Input: part model. Units: mm. Frame: model coordinates. Face numbers are marked on the shaded views. A direction names the side the tool comes from. Give positions to 0.01 mm unless a question says otherwise; leave off trailing zeros. Order: outer loops, then holes, each group sorted by start corner. A loop starts at its lowest first (then second) coordinate and runs counter-clockwise, first axis right, second up. Notation, with made-up numbers: (45, -27.5) - (61, -27.5) arc R21 cw to (61, 8.5) - close; hole circle Ø2 at (86.5, 63). An arc over 180 degrees is marked (long way). Answer in a Markdown table with one row per item. Add a question column.
1. Section query B-B on z = 6. Return loops of the section in (x, y).
2. Mould query, pull axis Z, two halves, no side actions, for the marked faces 1, 2 and 3. Classes: released by +Z, released by -Z, zero draft, split by the parting line, or undercut.
3. Section query D-D on x = 2.75. Return loops of the section in (y, z), and give its area (3 significant figures).
4. Contact query for flat-ended pins moving along their axis: pin 1 (5 mm diameter, centred on x = 4, y = -2.5, fed in from +Z); pin 2 (0.7 mm diameter, centred on x = 1, y = 14.5, fed in from +Z); pin 3 (3.5 mm diameter, centred on x = 12, z = 8.5, fed in from +Y). Output: stop coordinate, or through.
5. Ray query, line 1 (X direction, y = -8.25, z = 1.5); line 2 (Y direction, x = -13.5, z = 3); line 3 (Z direction, x = 6.25, y = 3.5). Return the intervals inside material, ascending. Write a range as [from, to].
6. Access query for the marked faces 4, 5 and 6. Directions: +Z, -Z, +X, -X, +Y, -Y. A direction counts if a zero-diameter tool reaches every point of the face in a straight line with its end or side. Return the directions, or none.
7. Section query C-C on y = -4. Return loops of the section in (x, z), and give its area (3 significant figures).
8. Section query A-A on z = 8.25. Return loops of the section in (x, y).
```python
from build123d import *

# Parameters (mm, degrees)
SKETCH1_W           = 30
SKETCH1_H           = 26
BOSS_EXTRUDE1_DEPTH = 10
CUT_EXTRUDE2_DEPTH  = 3.5
SKETCH3_W           = 3
SKETCH3_H           = 3
CUT_EXTRUDE3_DEPTH  = 3.5
SKETCH4_W           = 28
SKETCH4_H           = 23.6
CUT_EXTRUDE4_DEPTH  = 5.5
SKETCH5_W           = 3.7
SKETCH5_H           = 0.9
BOSS_EXTRUDE2_DEPTH = 1
SKETCH6_W           = 3.7
SKETCH6_H           = 0.9
BOSS_EXTRUDE3_DEPTH = 1


with BuildPart() as part:
    # Sketch1 → Boss-Extrude1 (new body)
    with BuildSketch(Plane.XY):
        with Locations((0.224911006, 2.218978102)):
            Rectangle(SKETCH1_W, SKETCH1_H)
    extrude(amount=BOSS_EXTRUDE1_DEPTH)

    # Sketch2 → Cut-Extrude2 (cut)
    with BuildSketch(Plane.XY.offset(10)):
        with BuildLine():
            Line((-13.775088994, 9.218978102), (-13.775088994, -4.781021898))
            ThreePointArc((-13.775088994, -4.781021898), (-12.896409337, -6.902342241), (-10.775088994, -7.781021898))
            Line((-10.775088994, -7.781021898), (-10.775088994, -10.781021898))
            Line((-10.775088994, -10.781021898), (11.224911006, -10.781021898))
            Line((11.224911006, -10.781021898), (11.224911006, -7.781021898))
            ThreePointArc((11.224911006, -7.781021898), (13.34623135, -6.902342241), (14.224911006, -4.781021898))
            Line((14.224911006, -4.781021898), (14.224911006, 9.218978102))
            ThreePointArc((14.224911006, 9.218978102), (13.34623135, 11.340298446), (11.224911006, 12.218978102))
            Line((11.224911006, 12.218978102), (11.224911006, 15.218978102))
            Line((11.224911006, 15.218978102), (-10.775088994, 15.218978102))
            Line((-10.775088994, 15.218978102), (-10.775088994, 12.218978102))
            ThreePointArc((-10.775088994, 12.218978102), (-12.896409337, 11.340298446), (-13.775088994, 9.218978102))
        make_face()
    extrude(amount=-CUT_EXTRUDE2_DEPTH, mode=Mode.SUBTRACT)

    # Sketch3 → Cut-Extrude3 (cut)
    with BuildSketch(Plane.XY.offset(10)):
        with Locations((-12.275088994, 13.718978102)):
            Rectangle(SKETCH3_W, SKETCH3_H)
        with Locations((12.724911006, -9.281021898)):
            Rectangle(SKETCH3_W, SKETCH3_H)
        with Locations((-12.275088994, -9.281021898)):
            Rectangle(SKETCH3_W, SKETCH3_H)
        with Locations((12.724911006, 13.718978102)):
            Rectangle(SKETCH3_W, SKETCH3_H)
    extrude(amount=-CUT_EXTRUDE3_DEPTH, mode=Mode.SUBTRACT)

    # Sketch4 → Cut-Extrude4 (cut)
    with BuildSketch(Plane.XY.offset(6.5)):
        with Locations((0.224911006, 2.218978102)):
            Rectangle(SKETCH4_W, SKETCH4_H)
    extrude(amount=-CUT_EXTRUDE4_DEPTH, mode=Mode.SUBTRACT)

    # Sketch5 → Boss-Extrude2 (add)
    with BuildSketch(Plane(origin=(0, 14.018978102, 0), x_dir=(-1, 0, 0), z_dir=(0, -1, 0))):
        with Locations((11.925088994, -6.05)):
            Rectangle(SKETCH5_W, SKETCH5_H)
        with Locations((-12.374911006, -6.05)):
            Rectangle(SKETCH5_W, SKETCH5_H)
    extrude(amount=BOSS_EXTRUDE2_DEPTH)

    # Sketch6 → Boss-Extrude3 (add)
    with BuildSketch(Plane(origin=(0, -9.581021898, 0), x_dir=(1, 0, 0), z_dir=(0, 1, 0))):
        with Locations((12.374911006, -6.05)):
            Rectangle(SKETCH6_W, SKETCH6_H)
        with Locations((-11.925088994, -6.05)):
            Rectangle(SKETCH6_W, SKETCH6_H)
    extrude(amount=BOSS_EXTRUDE3_DEPTH)


solid = part.part
```
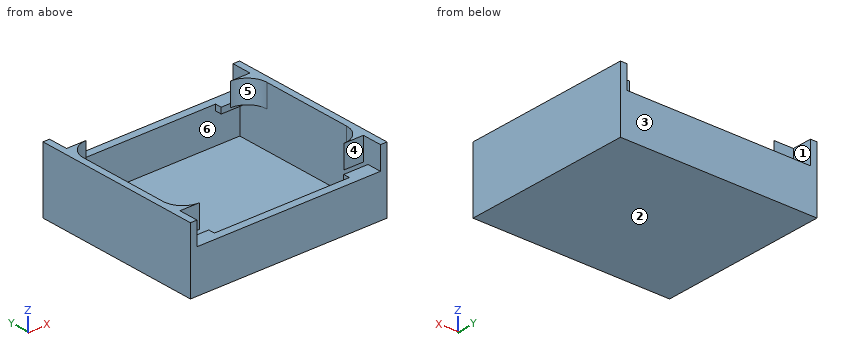
Answer:
| question | item | result |
|---|---|---|
| 1 | outline | (-14.78, -10.78) - (15.22, -10.78) - (15.22, 15.22) - (-14.78, 15.22) - close; hole (-13.78, -8.58) - (-10.08, -8.58) - (-10.08, -9.58) - (10.52, -9.58) - (10.52, -8.58) - (14.22, -8.58) - (14.22, 13.02) - (10.52, 13.02) - (10.52, 14.02) - (-10.08, 14.02) - (-10.08, 13.02) - (-13.78, 13.02) - close |
| 2 | face 1 | undercut |
| 2 | face 2 | released by -Z |
| 2 | face 3 | zero draft |
| 3 | outline | (-10.78, 0) - (15.22, 0) - (15.22, 6.5) - (14.02, 6.5) - (14.02, 1) - (-9.58, 1) - (-9.58, 6.5) - (-10.78, 6.5) - close |
| 3 | area | 39.2 mm² |
| 4 | pin 1 | stops at z = 1 |
| 4 | pin 2 | stops at z = 6.5 |
| 4 | pin 3 | stops at y = 12.22 |
| 5 | line 1 | x = [-14.78, -13.78], [14.22, 15.22] |
| 5 | line 2 | y = [-10.78, -9.58], [14.02, 15.22] |
| 5 | line 3 | z = [0, 1] |
| 6 | face 4 | +Z, -Y |
| 6 | face 5 | +Z |
| 6 | face 6 | none |
| 7 | outline | (-14.78, 0) - (15.22, 0) - (15.22, 10) - (14.22, 10) - (14.22, 1) - (-13.78, 1) - (-13.78, 10) - (-14.78, 10) - close |
| 7 | area | 48.0 mm² |
| 8 | outline | (-14.78, -10.78) - (-13.78, -10.78) - (-13.78, -7.78) - (-10.78, -7.78) arc R3 cw to (-13.78, -4.78) - (-13.78, 9.22) arc R3 cw to (-10.78, 12.22) - (-13.78, 12.22) - (-13.78, 15.22) - (-14.78, 15.22) - close; (11.22, -7.78) - (14.22, -7.78) - (14.22, -10.78) - (15.22, -10.78) - (15.22, 15.22) - (14.22, 15.22) - (14.22, 12.22) - (11.22, 12.22) arc R3 cw to (14.22, 9.22) - (14.22, -4.78) arc R3 cw to start |
